Part model, mm, in its own coordinate system. A direction names the side the tool comes from. Round coordinates to 2 decimals unless told otherwise and drop trailing zeros. Write each loop counter-clockwise with the first axis right and the second up, starting at its lowest first coordinate (ties: lowest second). Pieces come first, ordered by that corner, then holes.
1) Saw through at A-A on x = -0.5. Write the cut outline in (y, z).
2) Pull direction X, two halves, no side cores. Call faces 1 (the cylindrical face through (-21.45, 7.54, 1.74)), 2 (the flat face through (0.29, 0.195, 1.479)), 3 (the cylindrical face through (24.253, 2.168, 1.191)), 4 (the cylindrical face through (-24.253, 2.168, 1.191)): +X half, -X half, draft (parallel to the pull), parting line (faces both ways), or undercut.
3) Flat gauge pins, fed straight in: pin 1 (2 mm diameter, centred on y = 15.5, z = 1.5, fed in from +X); pin 2 (2 mm diameter, centred on x = -17.5, z = -2, fed in from +Y); pin 3 (3.5 mm diameter, centred on x = 0, y = 8.39, fed in from +Z); pin 4 (1.5 mm diameter, centred on x = 6.5, z = -3, fed in from +Y). Where does each tip first touch, or does it go through?
4) Saw through at C-C on z = 2.25. Count the separate pieces of the cut face and the enclosed holes in it, and give its area (3 significant figures).
5) Saw through at B-B on x = -20. Write the cut outline in (y, z), and give its area (3 significant figures).
6) Drill centre lines: L1, parallel to X at y = 5.5, z = 2.5; L2, parallel to X at y = 16.5, z = -0.75; L3, parallel to X at y = 29.5, z = -0.5. Where is each one in solid material? Low to high.
7) Which spindle directions (+Z, -Z, +X, -X, +Y, -Y) get a long thin tool onto all of the face, cutting with end or side? Do faces 5 (the cylindrical face through (-0.596, 27.936, -1.537)), 6 (the flat face through (9, 1.975, 1)), 7 (the flat face through (-5.316, 29.928, -0.093)). Say none if no direction does.
```python
from build123d import *

# Parameters (mm, degrees)
BOSS_EXTRUDE1_OUTLINE_R          = 1.575
BOSS_EXTRUDE1_OUTLINE_R_2        = 1.375
BOSS_EXTRUDE1_DEPTH              = 7.314466991
BOSS_EXTRUDE1_START              = 3
BOSS_EXTRUDE1_2_OUTLINE_W        = 26
BOSS_EXTRUDE1_2_OUTLINE_H        = 36
BOSS_EXTRUDE1_2_DEPTH            = 4.251890712
CBORE_FOR_M3_SHCS1_D             = 3.2
CBORE_FOR_M3_SHCS1_CBORE_D       = 6.5
CBORE_FOR_M3_SHCS1_CBORE_DEPTH   = 5.5
CBORE_FOR_M2_5_SHCS2_D           = 2.7
CBORE_FOR_M2_5_SHCS2_CBORE_D     = 5.5
CBORE_FOR_M2_5_SHCS2_CBORE_DEPTH = 3.5
CBORE_FOR_M2_5_SHCS1_D           = 2.7
CBORE_FOR_M2_5_SHCS1_CBORE_D     = 5.5
CBORE_FOR_M2_5_SHCS1_CBORE_DEPTH = 5
CUT_EXTRUDE2_DEPTH               = 43.124845356


with BuildPart() as part:
    # Boss-Extrude1: read off the stored shape, not the designer's step
    # Boss-Extrude1 outline → Boss-Extrude1 (new body)
    with BuildSketch(Plane(origin=(0, 0, 0), x_dir=(1, 0, 0), z_dir=(0, 0.13052619222005188, 0.9914448613738104))):
        with BuildLine():
            Line((0, 32.575), (0, 0))
            Line((0, 0), (20.75, 0))
            ThreePointArc((20.75, 0), (24.283668849, 2.045514976), (24.269768349, 6.128498422))
            Line((24.269768349, 6.128498422), (10.019768349, 30.553498422))
            ThreePointArc((10.019768349, 30.553498422), (8.529485024, 32.033668849), (6.5, 32.575))
            Line((6.5, 32.575), (0, 32.575))
        make_face()
        with Locations((20.75, 4.075)):
            Circle(BOSS_EXTRUDE1_OUTLINE_R, mode=Mode.SUBTRACT)
        with Locations((6.5, 28.5)):
            Circle(BOSS_EXTRUDE1_OUTLINE_R_2, mode=Mode.SUBTRACT)
    extrude(amount=BOSS_EXTRUDE1_DEPTH)

    # Boss-Extrude1 2 outline → Boss-Extrude1 2 (cut)
    with BuildSketch(Plane.XY.offset(BOSS_EXTRUDE1_START)):
        with Locations((13, 17)):
            Rectangle(BOSS_EXTRUDE1_2_OUTLINE_W, BOSS_EXTRUDE1_2_OUTLINE_H)
    extrude(amount=BOSS_EXTRUDE1_2_DEPTH, mode=Mode.SUBTRACT)

    # CBORE for M3 SHCS1 (through all)
    with Locations(Plane(origin=(0, 0.954729524, 7.251890712), x_dir=(-1, 0, 0), z_dir=(0, 0.1305261922200519, 0.9914448613738105))):
        with Locations((-20.75, -4.075)):
            CounterBoreHole(CBORE_FOR_M3_SHCS1_D / 2, CBORE_FOR_M3_SHCS1_CBORE_D / 2, CBORE_FOR_M3_SHCS1_CBORE_DEPTH)

    # CBORE for M2.5 SHCS2 (through all)
    with Locations(Plane(origin=(0, 0.954729524, 7.251890712), x_dir=(-1, 0, 0), z_dir=(0, 0.1305261922200519, 0.9914448613738105))):
        with Locations((-6.5, -28.5)):
            CounterBoreHole(CBORE_FOR_M2_5_SHCS2_D / 2, CBORE_FOR_M2_5_SHCS2_CBORE_D / 2, CBORE_FOR_M2_5_SHCS2_CBORE_DEPTH)

    # Mirror1: part across plane


with BuildPart() as part_1:
    add(part.part)
    add(part.part.mirror(Plane(origin=(0, 0, 0), x_dir=(0, 0, 1), z_dir=(1, 0, 0))))

    # CBORE for M2.5 SHCS1 (through all)
    with Locations(Plane(origin=(0, 0, -4.251890712), x_dir=(1, 0, 0), z_dir=(0, 0, -1))):
        with Locations((0, -25.251045884), (0, -8.394957493)):
            CounterBoreHole(CBORE_FOR_M2_5_SHCS1_D / 2, CBORE_FOR_M2_5_SHCS1_CBORE_D / 2, CBORE_FOR_M2_5_SHCS1_CBORE_DEPTH)

    # Sketch23 → Cut-Extrude2 (cut, through all)
    with BuildSketch(Plane.XY.offset(3)):
        with BuildLine():
            Line((12.623790508, 1.975153321), (4.480234369, 1.975153321))
            ThreePointArc((4.480234369, 1.975153321), (2.631634132, 3.211820389), (3.06913693, 5.392476156))
            ThreePointArc((3.06913693, 5.392476156), (4.328394301, 8.908169224), (2.397637796, 12.104730845))
            ThreePointArc((2.397637796, 12.104730845), (1.738647621, 12.826064632), (1.5, 13.773502121))
            Line((1.5, 13.773502121), (1.5, 17.985353527))
            ThreePointArc((1.5, 17.985353527), (3.063849532, 22.025225929), (6.940189675, 23.95918081))
            add(Edge.make_bspline(
                [(6.940189675, 23.95918081), (7.143604146, 23.981751029), (7.344683783, 24.016038635), (7.816288161, 24.124484553), (8.087087758, 24.209901876), (8.34862861, 24.315832383)],
                knots=[0.012994592, 0.012994592, 0.012994592, 0.012994592, 0.03125, 0.03125, 0.056300514, 0.056300514, 0.056300514, 0.056300514], degree=3))
            ThreePointArc((8.34862861, 24.315832383), (9.755972375, 24.375542014), (10.853622853, 23.492736744))
            Line((10.853622853, 23.492736744), (17.554812696, 12.149159325))
            ThreePointArc((17.554812696, 12.149159325), (17.723323038, 10.479170001), (16.560336213, 9.268913106))
            add(Edge.make_bspline(
                [(16.560336213, 9.268913106), (16.480857204, 9.196624751), (16.403239059, 9.122286883), (16.039402336, 8.755578367), (15.775927636, 8.431934638), (15.323177175, 7.748349007), (15.13178367, 7.387522034), (14.897329537, 6.817641357), (14.827739454, 6.621790337), (14.70905517, 6.227430948), (14.65970092, 6.02861076), (14.54474316, 5.446923453), (14.504405456, 5.059906471), (14.500341277, 4.666931627)],
                knots=[0.616779988, 0.616779988, 0.616779988, 0.616779988, 0.625, 0.625, 0.65625, 0.65625, 0.6875, 0.6875, 0.703125, 0.703125, 0.71875, 0.71875, 0.748473893, 0.748473893, 0.748473893, 0.748473893], degree=3))
            ThreePointArc((14.500341277, 4.666931627), (14.264454492, 2.831378127), (12.623790508, 1.975153321))
        make_face()
    cut_extrude2 = extrude(amount=-CUT_EXTRUDE2_DEPTH, mode=Mode.SUBTRACT)

    # Mirror2: Cut-Extrude2 across plane
    add(cut_extrude2.mirror(Plane(origin=(0, 0, 0), x_dir=(0, 0, 1), z_dir=(1, 0, 0))), mode=Mode.SUBTRACT)


solid = part_1.part
```
Completed:
1. outline: (0, 0) - (5.69, -0.75) - (5.69, 0.75) - (7.14, 0.75) - (7.14, 3) - (0.39, 3) - close; (9.65, 0.75) - (11.1, 0.75) - (11.1, -1.46) - (22.55, -2.97) - (22.55, 0.75) - (24, 0.75) - (24, 3) - (9.65, 3) - close; (26.51, 0.75) - (27.96, 0.75) - (27.96, -3.68) - (32.3, -4.25) - (33.25, 3) - (26.51, 3) - close
2. face 1: undercut
2. face 2: draft
2. face 3: +X half
2. face 4: -X half
3. pin 1: stops at x = 19.58
3. pin 2: stops at y = 19.36
3. pin 3: stops at z = 3
3. pin 4: stops at y = 32.56
4. separate pieces: 1
4. enclosed holes: 8
4. area: 525 mm2
5. outline: (0, 0) - (2.64, -0.35) - (2.88, 1.45) - (1.14, 1.68) - (1.32, 3) - (0.39, 3) - close; (5.44, -0.72) - (13.33, -1.76) - (13.96, 3) - (7.69, 3) - (7.41, 0.85) - (5.68, 1.08) - close
5. area: 36.4 mm2
6. L1: x = -24.69 to -23.83, -17.67 to -14.56, -3.17 to 3.17, 14.56 to 17.67, 23.83 to 24.69
6. L2: x = -18.24 to -14.98, -1.5 to 1.5, 14.98 to 18.24
6. L3: x = -10.74 to -7.61, -5.39 to 5.39, 7.61 to 10.74
7. face 5: -Z
7. face 6: +Z, -Z
7. face 7: none
